Geometry: see drawing. Coordinates: mm, zero at the bounding-box minimum. A direction names the side the tool comes from. Coordinates: 2 decimals unless noted, no trailing zeros. Order: outer loops, then holes, each group sorted by start corner. A loop starts at its lowest first (then second) coordinate and runs counter-clockwise, first axis right, second up. Notation, with made-up numbers: (60.5, -3.5) -> (95.5, -3.5) arc R8 ccw to (95.5, 1.5) -> close; hole circle Ø6 at (19, -22). An arc over 180 degrees is marked (long way). Use one line per item in the form item = value.
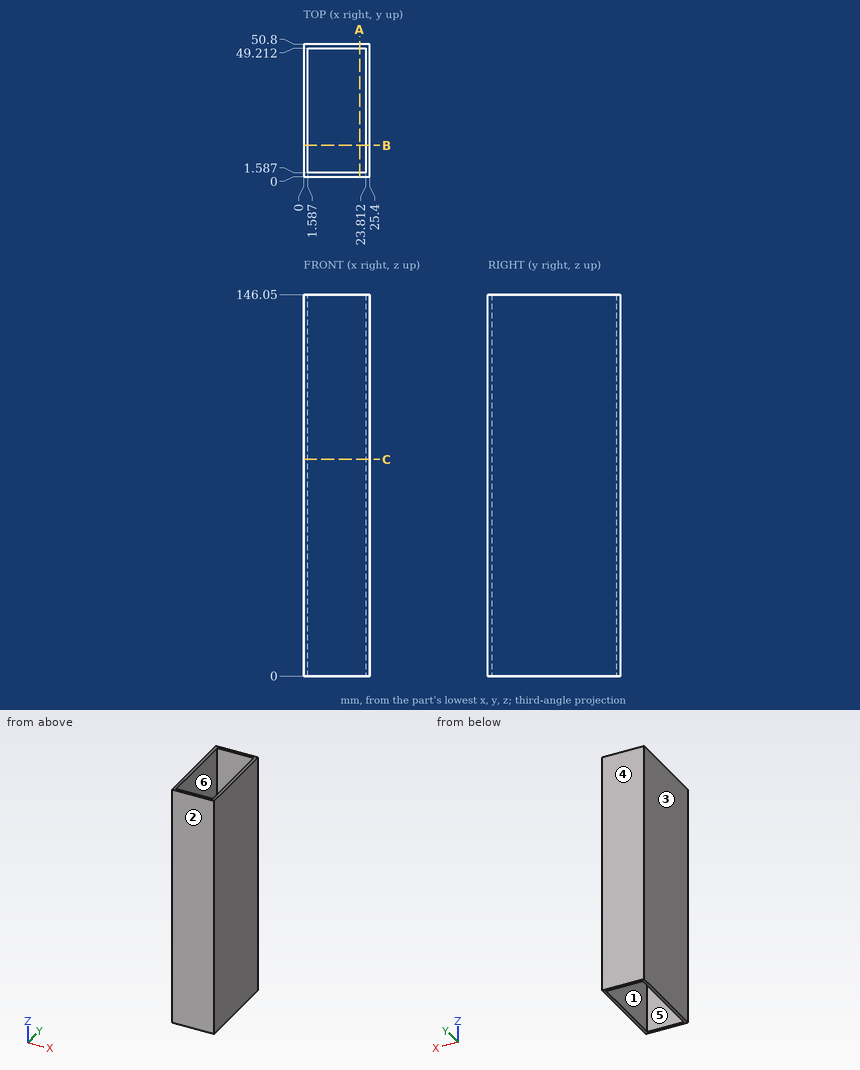
1) Section C-C, the plane z = 83. Output: boundary loops of the cut face in (x, y).
Results found:
outline = (0, 0) -> (25.4, 0) -> (25.4, 50.8) -> (0, 50.8) -> close; hole (1.59, 1.59) -> (23.81, 1.59) -> (23.81, 49.21) -> (1.59, 49.21) -> close
2) Pull-direction query (Y, two-part tool) for the marked faces 3, 4, 5 and 6; classes: released by +Y, released by -Y, zero draft, split by the parting line, or undercut.
Results found:
face_3 = zero draft
face_4 = released by +Y
face_5 = undercut
face_6 = undercut
3) Section A-A, the plane x = 21.5. Output: boundary loops of the cut face in (y, z).
Results found:
outline = (0, 0) -> (1.59, 0) -> (1.59, 146.05) -> (0, 146.05) -> close; (49.21, 0) -> (50.8, 0) -> (50.8, 146.05) -> (49.21, 146.05) -> close
4) Access query for the marked faces 1 and 2. Directions: +Z, -Z, +X, -X, +Y, -Y. A direction counts if a zero-diameter tool reaches every point of the face in a straight line with its end or side. Return the directions, or none.
Results found:
face_1 = +Z, -Z
face_2 = +Z, -Z, +X, -X, -Y
5) Material intervals for probe 1 along X at (y, z) = (23, 96); probe 2 along Y at (x, z) = (5.75, 54), sorted ascending. Write a range as from..to.
Results found:
probe_1 = 0..1.59, 23.81..25.4
probe_2 = 0..1.59, 49.21..50.8
6) Section B-B, the plane y = 12. Output: boundary loops of the cut face in (x, z).
Results found:
outline = (0, 0) -> (1.59, 0) -> (1.59, 146.05) -> (0, 146.05) -> close; (23.81, 0) -> (25.4, 0) -> (25.4, 146.05) -> (23.81, 146.05) -> close
